Source: CAD feature listing. Evaluate the final solid. Frame: model axes, mm. Round coordinates to 2 decimals unless told otherwise and drop trailing zeros. Order: outer loops, then holes, each group sorted by start corner. A loop starts at its lowest first (then second) coordinate and runs counter-clockwise, first axis right, second up. Notation, with made-up numbers: M 26.25,19 L 50.25,19 A24 cw 50.25,54 Z; hole C -16,-0.5 d3. An arc over 180 degrees is marked long. Use CSV: the item, a comma, the result in double quotes. Start each with the question number.
```python
from build123d import *

# Parameters (mm, degrees)
SKETCH1_R           = 63.5
SKETCH1_R_2         = 38.1
BOSS_EXTRUDE1_DEPTH = 19.05
SKETCH2_R           = 66.04
SKETCH2_R_2         = 38.1
BOSS_EXTRUDE2_DEPTH = 2.54
SCALE1_SCALE        = 0.111317254


with BuildPart() as part:
    # Sketch1 → Boss-Extrude1 (new body)
    with BuildSketch(Plane(origin=(0, 0, 0), x_dir=(0, 0, -1), z_dir=(1, 0, 0))):
        with Locations(Location((0, 0, 0), (0, 0, 180))):
            Circle(SKETCH1_R)
        with Locations(Location((0, 0, 0), (0, 0, 180))):
            Circle(SKETCH1_R_2, mode=Mode.SUBTRACT)
    extrude(amount=BOSS_EXTRUDE1_DEPTH)

    # Sketch2 → Boss-Extrude2 (add)
    with BuildSketch(Plane(origin=(19.05, 0, 0), x_dir=(0, 0, -1), z_dir=(1, 0, 0))):
        Circle(SKETCH2_R)
        with Locations(Location((0, 0, 0), (0, 0, 180))):
            Circle(SKETCH2_R_2, mode=Mode.SUBTRACT)
    extrude(amount=BOSS_EXTRUDE2_DEPTH)


with BuildPart() as part_1:
    # Scale1: scaled about (10.935763547, 0, 0)
    add(part.part.scale(SCALE1_SCALE).moved(Location((9.718424377, 0, 0))))


solid = part_1.part
```
(1) Line query: line 1 along Y through (x, z) = (11.15, 0); line 2 along X through (y, z) = (-4.5, -5.5); line 3 along Y through (x, z) = (10.5, 2.5). Output: solid intervals per line, ascending.
(2) Section A-A on z = 0. Return loops of the section in (x, y), plus the area to 3 significant figures.
(3) Section C-C on x = 10.4. Return loops of the section in (y, z), plus the area to 3 significant figures.
(4) Draft query along Y for faces 1 (the face through (10.76, 6.9, -1.53)), 2 (the face through (12.122, -3.2, -3.2)), 3 (the face through (11, 3, -3)). Return one class per face: pulls with the +Y half, pulls with the -Y half, needs draft (parallel to the pull), parting line crosses it, or undercut.
(5) Section D-D on y = -4.75. Return loops of the section in (x, z).
Results below:
1,line 1,"y = -7.07 to -4.24, 4.24 to 7.07"
1,line 2,"x = 11.84 to 12.12"
1,line 3,"y = -6.61 to -3.43, 3.43 to 6.61"
2,outline,"M 9.72,-7.07 L 11.84,-7.07 L 11.84,-7.35 L 12.12,-7.35 L 12.12,-4.24 L 9.72,-4.24 Z; M 9.72,4.24 L 12.12,4.24 L 12.12,7.35 L 11.84,7.35 L 11.84,7.07 L 9.72,7.07 Z"
2,area,"13.8 mm2"
3,outline,"C 0,0 d14.14; hole C 0,0 d8.48"
3,area,"100 mm2"
4,face 1,"parting line crosses it"
4,face 2,"needs draft"
4,face 3,"undercut"
5,outline,"M 9.72,-5.23 L 11.84,-5.23 L 11.84,-5.61 L 12.12,-5.61 L 12.12,5.61 L 11.84,5.61 L 11.84,5.23 L 9.72,5.23 Z"
